Verification items for the finished model (mm, model axes). Face numbers are marked on the shaded views. A direction names the side the tool comes from. Give positions to 0.01 mm unless a question says otherwise; leave off trailing zeros. Loops run counter-clockwise (first coordinate to the right, second up) from the corner with the lowest first, then second, coordinate; pieces in that order, holes last. Notation, with made-up numbers: (76.5, 9.25) -> (110.5, 9.25) arc R19 ccw to (110.5, 45.25) -> close; hole circle Ø11 at (81, 82). An arc over 180 degrees is marked (long way). Answer in a Markdown table with one row per item. Add a question column.
Q1. Release check for a two-part mould opening along Z. For the marked faces 1, 2 and 3 record: pulls with the +Z half, pulls with the -Z half, needs draft (parallel to the pull), parting line crosses it, or undercut.
Q2. Section check A-A on z = 0. Enter the section's corners in (x, y), and give its area (3 significant figures).
Q3. Section check B-B on x = 0. Enter the section's corners in (y, z).
Q4. Set-up check for the marked faces 4, 5, 6 and 7: record each of +Z, -Z, +X, -X, +Y, -Y from which the full face is reachable in a straight line by a thin tool's end or side.
Q5. Material ranges on probe 1 along Z at (x, y) = (0, 3.55); probe 2 along X at (y, z) = (5.75, 0.5); probe 3 along Y at (x, z) = (-11, 6), recorded low to high.
Q6. Gauge pin test, flat ends, axial feed: P1, Ø2.5, axis at x = -21, z = 9, coming from the -Y side; P2, Ø2, axis at x = -14, y = 15, coming from the +Z side; P3, Ø1, axis at x = -3, z = 13.5, coming from the +Y side; P4, Ø21, axis at x = 0, z = 0, coming from the -Y side. Record the tip position at first contact, or that the pin passes through.
```python
from build123d import *
from build123d.topology import SkipClean

# Parameters (mm, degrees)
SKETCH1_R           = 24
BOSS_EXTRUDE1_DEPTH = 18
HOLE2_D             = 24
HOLE2_DEPTH         = 18
HOLE2_CBORE_D       = 35
HOLE2_CBORE_DEPTH   = 12
HOLE2_TIP           = 7.210327428
CUT_EXTRUDE1_START  = -12
CUT_EXTRUDE1_DEPTH  = 12
SKETCH7_R           = 24
SKETCH7_R_2         = 21
CUT_EXTRUDE2_DEPTH  = 6
FILLET1_R           = 2


with BuildPart() as part:
    # Sketch1 → Boss-Extrude1 (new body)
    with BuildSketch(Plane(origin=(0, 0, 0), x_dir=(1, 0, 0), z_dir=(0, 1, 0))):
        with Locations(Location((0, 0, 0), (0, 0, 270))):
            Circle(SKETCH1_R)
    extrude(amount=BOSS_EXTRUDE1_DEPTH)

    # Hole2
    with Locations(Plane(origin=(0, 18, 0), x_dir=(1, 0, 0), z_dir=(0, 1, 0))):
        with Locations((0, 0)):
            CounterBoreHole(HOLE2_D / 2, HOLE2_CBORE_D / 2, HOLE2_CBORE_DEPTH, depth=HOLE2_DEPTH)
            with Locations((0, 0, -(HOLE2_DEPTH + HOLE2_TIP / 2))):  # 118° drill point
                Cone(0, HOLE2_D / 2, HOLE2_TIP, mode=Mode.SUBTRACT)

    # Sketch6 → Cut-Extrude1 (cut)
    with BuildSketch(Plane(origin=(0, 18, 0), x_dir=(1, 0, 0), z_dir=(0, 1, 0)).offset(CUT_EXTRUDE1_START)):
        with BuildLine():
            Line((20.784609691, 3), (23.8117618, 3))
            ThreePointArc((23.8117618, 3), (22.552622899, 8.20848344), (20.169230637, 13.00777212))
            Line((20.169230637, 13.00777212), (17.850297585, 11.061956252))
            ThreePointArc((17.850297585, 11.061956252), (19.733545037, 7.18242301), (20.784609691, 3))
        make_face()
        with BuildLine():
            Line((20.784609691, -3), (23.8117618, -3))
            ThreePointArc((23.8117618, -3), (22.552622899, -8.20848344), (20.169230637, -13.00777212))
            Line((20.169230637, -13.00777212), (17.850297585, -11.061956252))
            ThreePointArc((17.850297585, -11.061956252), (19.733545037, -7.18242301), (20.784609691, -3))
        make_face()
        with BuildLine():
            Line((13.993571927, -15.658222911), (16.312504978, -17.604038779))
            ThreePointArc((16.312504978, -17.604038779), (12, -20.784609691), (7.089292303, -22.9290631))
            Line((7.089292303, -22.9290631), (6.563632855, -19.947900234))
            ThreePointArc((6.563632855, -19.947900234), (10.5, -18.186533479), (13.993571927, -15.658222911))
        make_face()
        with BuildLine():
            Line((0.654786337, -20.9897893), (1.180445784, -23.970952166))
            ThreePointArc((1.180445784, -23.970952166), (-4.167556264, -23.635386072), (-9.307804688, -22.121590627))
            Line((-9.307804688, -22.121590627), (-7.794228634, -19.5))
            ThreePointArc((-7.794228634, -19.5), (-3.646611731, -20.680962813), (0.654786337, -20.9897893))
        make_face()
        with BuildLine():
            Line((-12.990381057, -16.5), (-14.503957111, -19.121590627))
            ThreePointArc((-14.503957111, -19.121590627), (-18.385066635, -15.426902632), (-21.349676421, -10.963180046))
            Line((-21.349676421, -10.963180046), (-18.505083922, -9.927833048))
            ThreePointArc((-18.505083922, -9.927833048), (-16.086933305, -13.498539803), (-12.990381057, -16.5))
        make_face()
        with BuildLine():
            Line((-20.557204782, -4.289677323), (-23.401797281, -5.325024321))
            ThreePointArc((-23.401797281, -5.325024321), (-24, 0), (-23.401797281, 5.325024321))
            Line((-23.401797281, 5.325024321), (-20.557204782, 4.289677323))
            ThreePointArc((-20.557204782, 4.289677323), (-21, 0), (-20.557204782, -4.289677323))
        make_face()
        with BuildLine():
            Line((-18.505083922, 9.927833048), (-21.349676421, 10.963180046))
            ThreePointArc((-21.349676421, 10.963180046), (-18.385066635, 15.426902632), (-14.503957111, 19.121590627))
            Line((-14.503957111, 19.121590627), (-12.990381057, 16.5))
            ThreePointArc((-12.990381057, 16.5), (-16.086933305, 13.498539803), (-18.505083922, 9.927833048))
        make_face()
        with BuildLine():
            Line((-7.794228634, 19.5), (-9.307804688, 22.121590627))
            ThreePointArc((-9.307804688, 22.121590627), (-4.167556264, 23.635386072), (1.180445784, 23.970952166))
            Line((1.180445784, 23.970952166), (0.654786337, 20.9897893))
            ThreePointArc((0.654786337, 20.9897893), (-3.646611731, 20.680962813), (-7.794228634, 19.5))
        make_face()
        with BuildLine():
            Line((6.563632855, 19.947900234), (7.089292303, 22.9290631))
            ThreePointArc((7.089292303, 22.9290631), (12, 20.784609691), (16.312504978, 17.604038779))
            Line((16.312504978, 17.604038779), (13.993571927, 15.658222911))
            ThreePointArc((13.993571927, 15.658222911), (10.5, 18.186533479), (6.563632855, 19.947900234))
        make_face()
    extrude(amount=CUT_EXTRUDE1_DEPTH, mode=Mode.SUBTRACT)

    # Sketch7 → Cut-Extrude2 (cut)
    with SkipClean():  # the faces are left unmerged after this step: merging them gives an invalid solid
        with BuildSketch(Plane.XZ):
            Circle(SKETCH7_R)
            with Locations(Location((0, 0, 0), (0, 0, 88.213210702))):
                Circle(SKETCH7_R_2, mode=Mode.SUBTRACT)
        extrude(amount=-CUT_EXTRUDE2_DEPTH, mode=Mode.SUBTRACT)

    # Fillet1
    fillet1_edges = [part.edges().sort_by_distance(p)[0] for p in [
        (-0.654786337, 0, -20.9897893),
    ]]
    fillet(fillet1_edges, radius=FILLET1_R)


solid = part.part
```
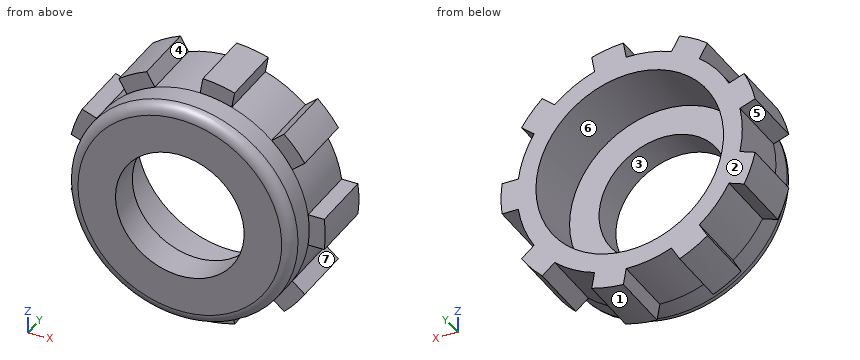
Taken from the geometry:
| question | item | result |
|---|---|---|
| 1 | face 1 | pulls with the -Z half |
| 1 | face 2 | needs draft |
| 1 | face 3 | undercut |
| 2 | outline | (-21, 2) arc R2 ccw to (-19, 0) -> (-12, 0) -> (-12, 6) -> (-17.5, 6) -> (-17.5, 18) -> (-21, 18) -> close; (12, 0) -> (19, 0) arc R2 ccw to (21, 2) -> (21, 6) -> (24, 6) -> (24, 18) -> (17.5, 18) -> (17.5, 6) -> (12, 6) -> close |
| 2 | area | 226 mm² |
| 3 | outline | (0, -19) arc R2 ccw to (2, -21) -> (18, -21) -> (18, -17.5) -> (6, -17.5) -> (6, -12) -> (0, -12) -> close; (0, 12) -> (6, 12) -> (6, 17.5) -> (18, 17.5) -> (18, 21) -> (2, 21) arc R2 ccw to (0, 19) -> close |
| 4 | face 4 | +Z, +Y, -Y |
| 4 | face 5 | -X, +Y, -Y |
| 4 | face 6 | +Y |
| 4 | face 7 | +X, +Y, -Y |
| 5 | probe 1 | z = -21 to -12, 12 to 21 |
| 5 | probe 2 | x = -20.99 to -11.99, 11.99 to 20.99 |
| 5 | probe 3 | y = 0 to 6 |
| 6 | P1 | stops at y = 6 |
| 6 | P2 | stops at z = 20.17 |
| 6 | P3 | stops at y = 6 |
| 6 | P4 | passes through |
